For this review, take the finished solid that the model builds, in its own axes (mm). Face numbers are marked on the shaded views. A direction names the side the tool comes from. Coordinates: 2 decimals unless noted, no trailing zeros. Order: outer loops, then holes, each group sorted by start corner. A loop starts at its lowest first (then second) coordinate and runs counter-clockwise, first axis right, second up. Notation, with made-up numbers: (-0.75, -38.5) -> (25.25, -38.5) arc R14 ccw to (25.25, -33.5) -> close; hole circle Ø2 at (-32.75, 52.5). An arc over 180 degrees is marked (long way). Return JSON: item names as keys, results as strings. Group by question number.
Item 1: Insertion check: pin 1 (1.5 mm diameter, centred on x = 3.5, y = 0, fed in from -Z); pin 2 (5 mm diameter, centred on x = 9, z = -3.5, fed in from -Y); pin 3 (4 mm diameter, centred on x = 9, y = -1.5, fed in from +Z). Each pin has a flat end and moves straight along its axis. Give the tip position at first contact, or say it passes through.
Item 2: For line 1 along X through (y, z) = (-3.5, -1.5); line 2 along Z through (x, y) = (2, 0); line 3 along Y through (x, z) = (7.5, 0), list the stretches that pass through material, from the lowest coordinate up.
Item 3: Machinability: for the marked faces 5 and 6, which of the approach directions +Z, -Z, +X, -X, +Y, -Y give a long, thin tool a straight path to every point of the face, cutting with its end or side? Answer none if there is none.
Item 4: Draft analysis for pull direction Z (two halves, no side actions). For the marked faces 1, 2, 3 and 4, state which applies: +Z half, -Z half, draft (parallel to the pull), parting line (faces both ways), or undercut.
Item 5: Take a section at A-A (x = 10.75). Write out the cut boundary in (y, z), then the cut area to 3 significant figures.
```python
from build123d import *

# Parameters (mm, degrees)
FILLET1_R    = 1
SKETCH3_W    = 1.03
SKETCH3_H    = 4.4
SKETCH4_W    = 1.03
SKETCH4_H    = 1.897120414
RECPAT_COUNT = 2
RECPAT_ANGLE = 90


with BuildPart() as part:
    # BodySke → Base-Revolve (revolve)
    with BuildSketch(Plane.XY):
        Polygon((0, 0), (0, 4.2), (0.5, 4.2), (2.7, 2), (12, 2), (12, 0), align=None)
    revolve(axis=Axis((-6.35, 0, 0), (1, 0, 0)))

    # Fillet1
    fillet1_edges = [part.edges().sort_by_distance(p)[0] for p in [
        (2.7, -2, 0),
    ]]
    fillet(fillet1_edges, radius=FILLET1_R)

    # Sketch3 → Recess section 0
    with BuildSketch(Plane.ZY):
        Rectangle(SKETCH3_W, SKETCH3_H)
    # Sketch4 → Recess section 1
    with BuildSketch(Plane.ZY.offset(-2.51)):
        Rectangle(SKETCH4_W, SKETCH4_H)
    recess = loft(mode=Mode.SUBTRACT)

    # RecPat: Recess ×2 about axis
    recpat_axis = Axis((0, 0, 0), (1, 0, 0))
    for i in range(1, RECPAT_COUNT):
        add(recess.rotate(recpat_axis, i * RECPAT_ANGLE / (RECPAT_COUNT - 1)), mode=Mode.SUBTRACT)

    # RecCorSke → RecessCore (revolve, cut)
    with BuildSketch(Plane.XY):
        Polygon((0, 0), (0, 1.026516298), (2.51, 0.851), (2.786506661, 0), align=None)
    revolve(axis=Axis((-3.175, 0, 0), (1, 0, 0)), mode=Mode.SUBTRACT)


solid = part.part
```
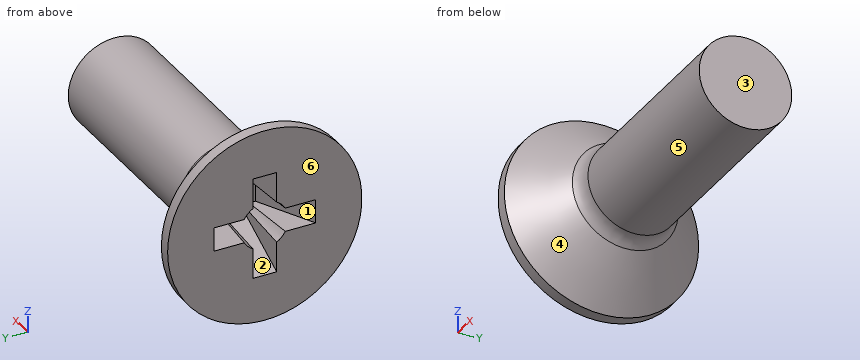
Findings below:
{
 "1": {"pin 1": "stops at z = -2.07", "pin 2": "stops at y = -1.73", "pin 3": "stops at z = 2"},
 "2": {"line 1": "x = 0 to 0.89", "line 2": "z = -2.7 to -1.2, 1.2 to 2.7", "line 3": "y = -2 to 2"},
 "3": {"face 5": "+X", "face 6": "+Z, -Z, -X, +Y, -Y"},
 "4": {"face 1": "undercut", "face 2": "undercut", "face 3": "draft", "face 4": "parting line"},
 "5": {"outline": "circle Ø4 at (0, 0)", "area": "12.6 mm2"}
}
